Answer from the drawing. Dimensions are ordinates in mm from the lowest x, y and z of the part. A direction names the side the tool comes from. Round coordinates to 2 decimals unless told otherwise and drop trailing zeros. Loops run counter-clockwise (first coordinate to the right, second up) from the corner with the lowest first, then second, coordinate; pieces in that order, holes last.
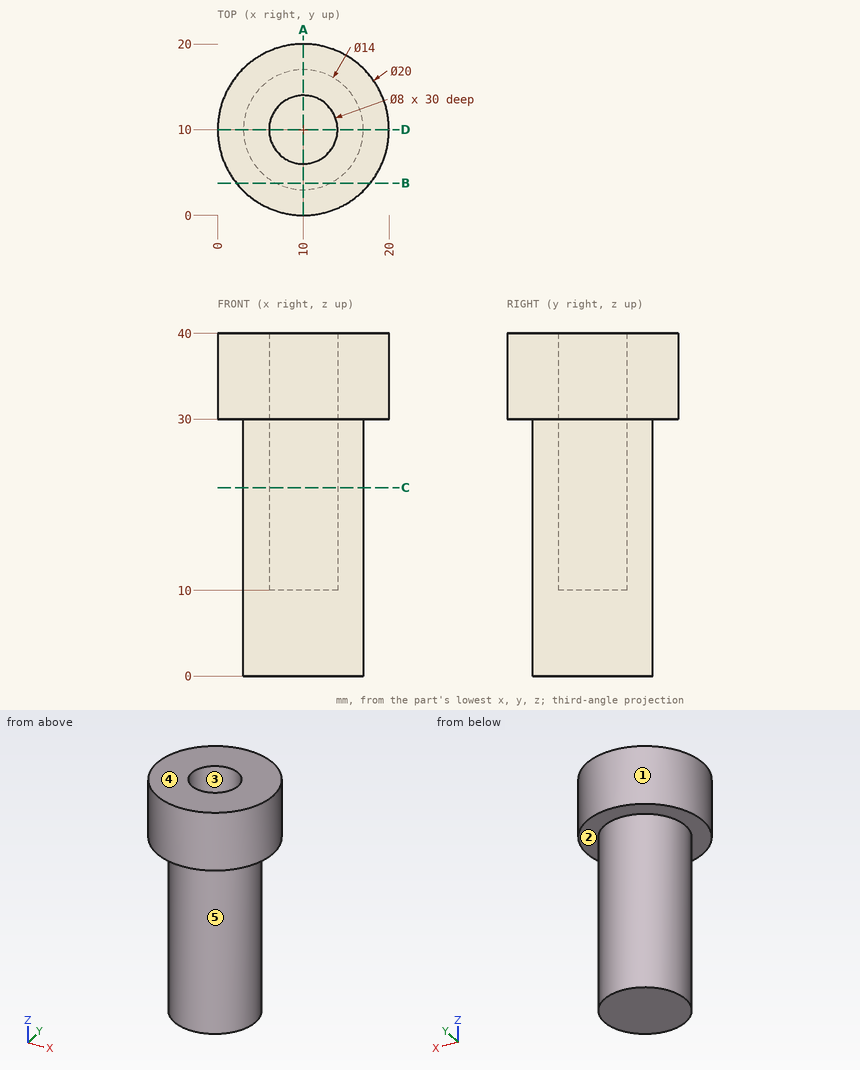
1. Find section A-A (x = 10). Write down the section's boundary in (y, z), then the cut area to 3 significant figures.
Answer key:
outline: (0, 30) - (3, 30) - (3, 0) - (17, 0) - (17, 30) - (20, 30) - (20, 40) - (14, 40) - (14, 10) - (6, 10) - (6, 40) - (0, 40) - close
area: 380 mm2
2. Consider probe 1 along Y at (x, z) = (10, 32.75); probe 2 along Z at (x, y) = (8.75, 7.5); probe 3 along Z at (x, y) = (9.25, 18.25). Determine where each line is inside the solid, lowest interval first.
Answer key:
probe 1: y = 0 to 6, 14 to 20
probe 2: z = 0 to 10
probe 3: z = 30 to 40
3. Given pin 1 (10.5 mm diameter, centred on x = 10, y = 10, fed in from -Z); pin 2 (8 mm diameter, centred on y = 16, z = 7.5, fed in from +X); pin 3 (1 mm diameter, centred on x = 8, z = 30.5, fed in from -Y); pin 4 (2 mm diameter, centred on x = 16, z = 11, fed in from +Y), each flat-ended and moving along its own axis, determine where each tip first touches the part or whether it passes through.
Answer key:
pin 1: stops at z = 0
pin 2: stops at x = 16.71
pin 3: stops at y = 0.11
pin 4: stops at y = 14.9
4. Find section B-B (y = 3.75). Write down the section's boundary in (x, z).
Answer key:
outline: (2.19, 30) - (6.85, 30) - (6.85, 0) - (13.15, 0) - (13.15, 30) - (17.81, 30) - (17.81, 40) - (2.19, 40) - close
5. Find section C-C (z = 22). Write down the section's boundary in (x, y).
Answer key:
outline: circle Ø14 at (10, 10); hole circle Ø8 at (10, 10)
6. Determine the mould class of the marked faces 3, 4 and 5 for opening direction Y: +Y half, -Y half, draft (parallel to the pull), parting line (faces both ways), or undercut.
Answer key:
face 3: undercut
face 4: draft
face 5: parting line
7. Which of the six approach directions +Z, -Z, +X, -X, +Y, -Y give full straight-line access (tool end or side, diameter ignored) to the marked faces 1 and 2?
Answer key:
face 1: +Z, -Z
face 2: -Z
